Study the drawing (mm; zero at the part's minimum x, y, z) and answer. A direction names the side the tool comes from. Give positions to 0.01 mm unless a question says otherwise; leave off trailing zeros. Order: outer loops, then holes, each group sorted by start corner. A loop starts at its lowest first (then second) coordinate and runs counter-clockwise, first axis right, second up. Notation, with made-up numbers: (42.5, -23) - (67.5, -23) arc R19 ccw to (67.5, -9) - close; hole circle Ø10 at (32, -19). An arc over 180 degrees is marked (long way). Write each question's results on one line, items separated by ' | '. Start each with the question number.
Q1. Find section B-B on x = 10.5. Give the vertices of the cut face in (y, z), and give its area (4 significant figures).
Q2. Find section C-C on y = 5. Give the vertices of the cut face in (x, z) (3 decimals).
Q3. For a pull along X with two mould halves and no side action, classify the marked faces 5, 6 and 7 as +X half, -X half, draft (parallel to the pull), parting line (faces both ways), or undercut.
Q4. Flat-ended cylindrical pins translate along their axes: P1, Ø1.9, axis at x = 10.5, z = 11.5, coming from the +Y side; P2, Ø1, axis at y = 6.5, z = 12.5, coming from the +X side; P3, Ø4.5, axis at x = 11.5, y = 6, coming from the -Z side; P4, Ø2, axis at y = 6, z = 9, coming from the -X side. Find the tip coordinate at first contact, or state that the pin passes through.
Q5. A tool of negligible diameter and unlimited length cuts with its end or side. For the marked faces 1, 2, 3 and 4, from which of +Z, -Z, +X, -X, +Y, -Y can it reach the whole face along a straight path? Write none if from no direction.
Q6. Find the intervals of material crossed by line 1 along Z through (x, y) = (10.5, 4.25); line 2 along X through (y, z) = (4.25, 23.75); line 3 along X through (y, z) = (1.5, 23.75), in increasing order. Write a range as from..to.
Q7. Find section D-D on y = 1.5. Give the vertices of the cut face in (x, z), and give its area (3 significant figures).
Q8. Find section A-A on z = 23.75. Give the vertices of the cut face in (x, y), and give its area (3 significant figures).
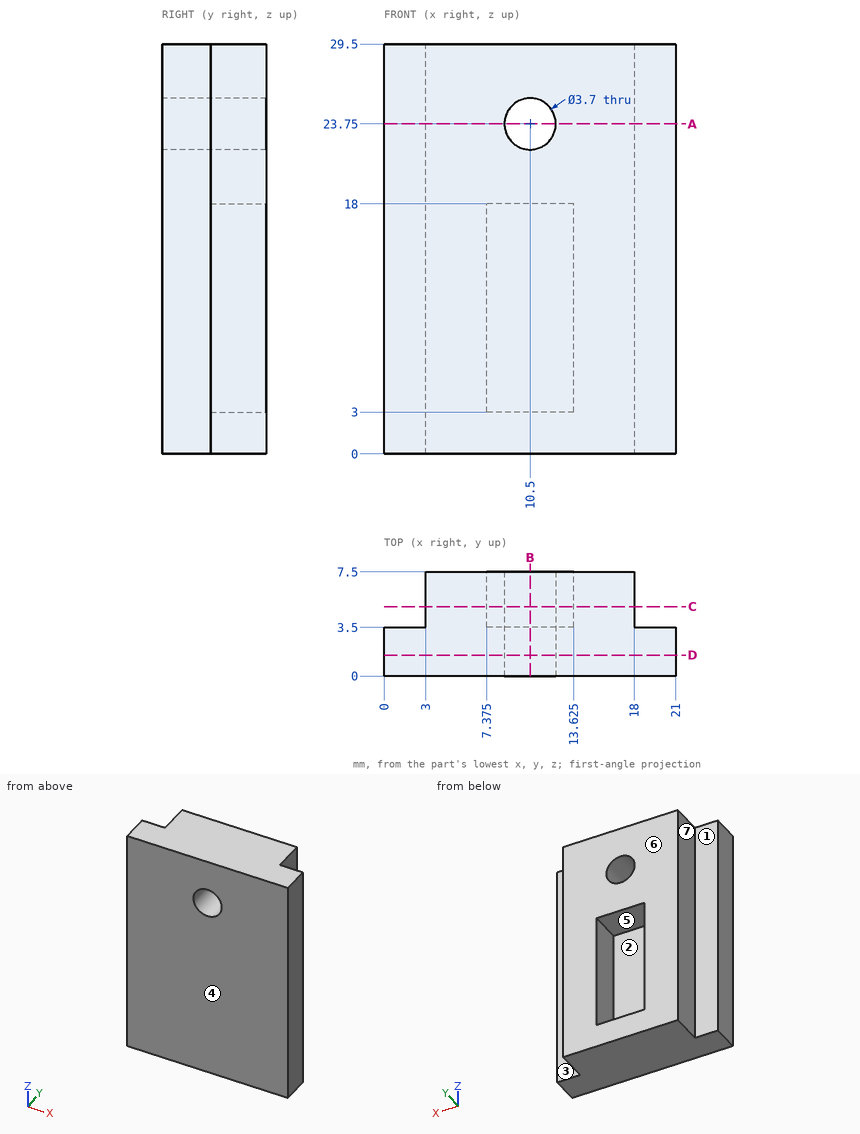
Working result:
1) outline: (0, 0) - (7.5, 0) - (7.5, 3) - (3.5, 3) - (3.5, 18) - (7.5, 18) - (7.5, 21.9) - (0, 21.9) - close; (0, 25.6) - (7.5, 25.6) - (7.5, 29.5) - (0, 29.5) - close | area: 133.5 mm²
2) outline: (3, 0) - (18, 0) - (18, 29.5) - (3, 29.5) - close; hole (7.375, 3) - (13.625, 3) - (13.625, 18) - (7.375, 18) - close; hole circle Ø3.7 at (10.5, 23.75)
3) face 5: undercut | face 6: draft | face 7: -X half
4) P1: y = 3.5 | P2: x = 18 | P3: z = 0 | P4: x = 3
5) face 1: +Z, -Z, -X, +Y | face 2: +Y | face 3: +Z, -Z, +X, +Y | face 4: +Z, -Z, +X, -X, -Y
6) line 1: 0..3, 18..21.9, 25.6..29.5 | line 2: 3..8.65, 12.35..18 | line 3: 0..8.65, 12.35..21
7) outline: (0, 0) - (21, 0) - (21, 29.5) - (0, 29.5) - close; hole circle Ø3.7 at (10.5, 23.75) | area: 609 mm²
8) outline: (0, 0) - (8.65, 0) - (8.65, 7.5) - (3, 7.5) - (3, 3.5) - (0, 3.5) - close; (12.35, 0) - (21, 0) - (21, 3.5) - (18, 3.5) - (18, 7.5) - (12.35, 7.5) - close | area: 106 mm²
